Read the model definition and answer for the solid it produces. Units are mm, in the model's axes. A direction names the side the tool comes from. Round coordinates to 2 decimals unless told otherwise and drop trailing zeros. Loops run counter-clockwise (first coordinate to the right, second up) from the corner with the lowest first, then second, coordinate; pieces in that order, holes last. Notation, with made-up numbers: (21.5, -11.5) - (63.5, -11.5) arc R17 ccw to (63.5, -3.5) - close; hole circle Ø2 at (36.5, 74). An arc over 180 degrees is marked (long way). Use one line per item in the form item = value. Start each with the question number.
```python
from build123d import *

# Parameters (mm, degrees)
BOSS_EXTRUDE1_DEPTH      = 11
BOSS_EXTRUDE1_DEPTH_BACK = 5
SKETCH1_R                = 15
SKETCH1_R_2              = 13
BOSS_EXTRUDE2_DEPTH      = 5
BOSS_EXTRUDE2_DEPTH_BACK = 10
SKETCH2_R                = 23
SKETCH2_R_2              = 8.75
SKETCH6_R                = 1.5
CUT_EXTRUDE1_DEPTH       = 23
CUT_EXTRUDE2_DEPTH       = 1.25
CUT_EXTRUDE2_DEPTH_BACK  = 1.25
SKETCH13_R               = 13
SKETCH13_R_2             = 8.75
BOSS_EXTRUDE5_DEPTH      = 6
SKETCH14_R               = 12
SKETCH14_R_2             = 8.75
BOSS_EXTRUDE6_DEPTH      = 16
BOSS_EXTRUDE7_START      = 20
SKETCH17_R               = 11
SKETCH17_R_2             = 8.75
BOSS_EXTRUDE7_DEPTH      = 20
CUT_EXTRUDE3_DEPTH       = 57
CUT_EXTRUDE3_DEPTH_BACK  = 57
SKETCH18_R               = 1.5
SKETCH19_R               = 3
CUT_EXTRUDE4_DEPTH       = 14
BOSS_EXTRUDE8_START      = 6
SKETCH20_R               = 23
SKETCH20_R_2             = 11
BOSS_EXTRUDE8_DEPTH      = 6


with BuildPart() as part:
    # Sketch1 → Boss-Extrude1 (new, two sides: drawn at the far end of the back side and taken through both)
    with BuildSketch(Plane.XY.offset(-BOSS_EXTRUDE1_DEPTH_BACK)):
        Circle(SKETCH1_R)
        Circle(SKETCH1_R_2, mode=Mode.SUBTRACT)
    extrude(amount=BOSS_EXTRUDE1_DEPTH + BOSS_EXTRUDE1_DEPTH_BACK)

    # Sketch2 → Boss-Extrude2 (add, two sides: drawn at the far end of the back side and taken through both)
    with BuildSketch(Plane.XY.offset(-BOSS_EXTRUDE2_DEPTH_BACK)):
        Circle(SKETCH2_R)
        Circle(SKETCH2_R_2, mode=Mode.SUBTRACT)
    extrude(amount=BOSS_EXTRUDE2_DEPTH + BOSS_EXTRUDE2_DEPTH_BACK)

    # Sketch6 → Cut-Extrude1 (cut)
    with BuildSketch(Plane.XY.offset(5)):
        with Locations((0, 19)):
            Circle(SKETCH6_R)
        with Locations((19, 0)):
            Circle(SKETCH6_R)
        with Locations((0, -19)):
            Circle(SKETCH6_R)
        with Locations((-19, 0)):
            Circle(SKETCH6_R)
    extrude(amount=-CUT_EXTRUDE1_DEPTH, mode=Mode.SUBTRACT)

    # Sketch9 → Cut-Extrude2 (cut, two sides: drawn at the far end of the back side and taken through both)
    with BuildSketch(Plane.XY.offset(-CUT_EXTRUDE2_DEPTH_BACK)):
        Polygon((-2.8, 20.616580754), (-2.8, 26.448707706), (2.8, 26.448707706), (2.8, 20.616580754), (2.8, 17.383419246), (0, 15.766838493), (-2.8, 17.383419246), align=None)
        Polygon((20.616580754, 2.8), (26.448707706, 2.8), (26.448707706, -2.8), (20.616580754, -2.8), (17.383419246, -2.8), (15.766838493, 0), (17.383419246, 2.8), align=None)
        Polygon((2.8, -20.616580754), (2.8, -26.448707706), (-2.8, -26.448707706), (-2.8, -20.616580754), (-2.8, -17.383419246), (0, -15.766838493), (2.8, -17.383419246), align=None)
        Polygon((-20.616580754, -2.8), (-26.448707706, -2.8), (-26.448707706, 2.8), (-20.616580754, 2.8), (-17.383419246, 2.8), (-15.766838493, 0), (-17.383419246, -2.8), align=None)
    extrude(amount=CUT_EXTRUDE2_DEPTH + CUT_EXTRUDE2_DEPTH_BACK, mode=Mode.SUBTRACT)

    # Sketch13 → Boss-Extrude5 (add)
    with BuildSketch(Plane.XY.offset(5)):
        Circle(SKETCH13_R)
        Circle(SKETCH13_R_2, mode=Mode.SUBTRACT)
    extrude(amount=BOSS_EXTRUDE5_DEPTH)

    # Sketch14 → Boss-Extrude6 (add)
    with BuildSketch(Plane.XY.offset(11)):
        Circle(SKETCH14_R)
        Circle(SKETCH14_R_2, mode=Mode.SUBTRACT)
    extrude(amount=BOSS_EXTRUDE6_DEPTH)

    # Sketch17 → Boss-Extrude7 (add)
    with BuildSketch(Plane(origin=(0, 0, -10), x_dir=(-1, 0, 0), z_dir=(0, 0, -1)).offset(BOSS_EXTRUDE7_START)):
        with Locations(Location((0, 0, 0), (0, 0, 180))):
            Circle(SKETCH17_R)
        with Locations(Location((0, 0, 0), (0, 0, 180))):
            Circle(SKETCH17_R_2, mode=Mode.SUBTRACT)
    extrude(amount=-BOSS_EXTRUDE7_DEPTH)

    # Sketch18 → Cut-Extrude3 (cut, two sides: drawn at the far end of the back side and taken through both)
    with BuildSketch(Plane(origin=(0, 0, 0), x_dir=(0, 0, -1), z_dir=(1, 0, 0)).offset(-CUT_EXTRUDE3_DEPTH_BACK)):
        with Locations(Location((-22, 0, 0), (0, 0, 180))):
            Circle(SKETCH18_R)
    extrude(amount=CUT_EXTRUDE3_DEPTH + CUT_EXTRUDE3_DEPTH_BACK, mode=Mode.SUBTRACT)

    # Sketch19 → Cut-Extrude4 (cut)
    with BuildSketch(Plane(origin=(10.25, 0, 0), x_dir=(0, 0, -1), z_dir=(1, 0, 0))):
        with Locations((-22, 0)):
            Circle(SKETCH19_R)
    cut_extrude4 = extrude(amount=CUT_EXTRUDE4_DEPTH, mode=Mode.SUBTRACT)

    # Mirror1: Cut-Extrude4 across plane
    add(cut_extrude4.mirror(Plane(origin=(0, 0, 0), x_dir=(0, 0, 1), z_dir=(1, 0, 0))), mode=Mode.SUBTRACT)

    # Sketch20 → Boss-Extrude8 (add)
    with BuildSketch(Plane(origin=(0, 0, -10), x_dir=(-1, 0, 0), z_dir=(0, 0, -1)).offset(BOSS_EXTRUDE8_START)):
        with Locations(Location((0, 0, 0), (0, 0, 180))):
            Circle(SKETCH20_R)
        Circle(SKETCH20_R_2, mode=Mode.SUBTRACT)
    extrude(amount=-BOSS_EXTRUDE8_DEPTH)


solid = part.part
```
1) A cutting plane is placed at A-A on x = -5. Write down the section's boundary in (y, z).
2) Determine the mould class of faces 6 (the flat face through (10, -5, -16)), 7 (the cylindrical face through (-14.985, 0.66, 7.958)), 8 (the flat face through (16.564, 1.38, -0.018)), 9 (the cylindrical face through (11.11, -1.15, 19.23)) for opening direction Y: +Y half, -Y half, draft (parallel to the pull), parting line (faces both ways), or undercut.
3) A cutting plane is placed at D-D on z = -23. Write down the section's boundary in (x, y), plus the area to 3 significant figures.
4) A cutting plane is placed at C-C on y = 8. Write down the section's boundary in (x, z).
5) A cutting plane is placed at B-B on z = 22. Write down the section's boundary in (x, y), plus the area to 3 significant figures.
6) For faces 1 (the flat face through (-1.38, 16.564, -0.018)), 2 (the flat face through (0, -21, 1.25)), 3 (the cylindrical face through (-0.195, 20.487, 3.151)), 4 (the flat face through (20, -2.8, 0)), 5 (the cylindrical face through (-11.12, -1.15, 19.23)), determine the directions among +Z, -Z, +X, -X, +Y, -Y from which every point of the face is accessible in a straight line to the end or side of a thin tool.
7) Flat-ended cylindrical pins translate along their axes: pin 1 (3.5 mm diameter, centred on x = 0.5, y = -19.5, fed in from +Z); pin 2 (3 mm diameter, centred on y = 1.5, z = 23.5, fed in from +X); pin 3 (1.8 mm diameter, centred on x = 0, y = 19, fed in from +Z); pin 4 (2 mm diameter, centred on y = -0.5, z = -2.5, fed in from -X). Find the tip coordinate at first contact, or state that the pin passes through.
8) Straight lines are drawn through the part: line 1 (Z direction, x = 2.5, y = 18.5); line 2 (Z direction, x = 18.5, y = 3); line 3 (Y direction, x = -7.5, z = 17). For each, find the intervals that lie inside material, in ascending order. Write a range as from..to.
Checks:
q1.outline = (-22.45, -16) - (-9.8, -16) - (-9.8, -30) - (-7.18, -30) - (-7.18, 27) - (-10.91, 27) - (-10.91, 11) - (-14.14, 11) - (-14.14, 5) - (-22.45, 5) - close; (7.18, -30) - (9.8, -30) - (9.8, -16) - (22.45, -16) - (22.45, 5) - (14.14, 5) - (14.14, 11) - (10.91, 11) - (10.91, 27) - (7.18, 27) - close
q2.face_6 = draft
q2.face_7 = parting line
q2.face_8 = undercut
q2.face_9 = undercut
q3.outline = circle Ø22 at (0, 0); hole circle Ø17.5 at (0, 0)
q3.area = 140 mm²
q4.outline = (-21.56, -16) - (-7.55, -16) - (-7.55, -30) - (-3.54, -30) - (-3.54, 27) - (-8.94, 27) - (-8.94, 11) - (-12.69, 11) - (-12.69, 5) - (-21.56, 5) - close; (3.54, -30) - (7.55, -30) - (7.55, -16) - (21.56, -16) - (21.56, 5) - (12.69, 5) - (12.69, 11) - (8.94, 11) - (8.94, 27) - (3.54, 27) - close
q5.outline = (-11.62, -3) arc R12 ccw to (11.62, -3) - (10.25, -3) - (10.25, -1.5) - (8.62, -1.5) arc R8.75 cw to (-8.62, -1.5) - (-10.25, -1.5) - (-10.25, -3) - close; (-11.62, 3) - (-10.25, 3) - (-10.25, 1.5) - (-8.62, 1.5) arc R8.75 cw to (8.62, 1.5) - (10.25, 1.5) - (10.25, 3) - (11.62, 3) arc R12 ccw to start
q5.area = 183 mm²
q6.face_1 = +Y
q6.face_2 = -Y
q6.face_3 = +Z
q6.face_4 = +X
q6.face_5 = -X
q7.pin_1 = 5
q7.pin_2 = 11.97
q7.pin_3 = -10
q7.pin_4 = -23
q8.line_1 = -16..-1.25, 1.25..5
q8.line_2 = -16..5
q8.line_3 = -9.37..-4.51, 4.51..9.37
